Part model, mm, in its own coordinate system. A direction names the side the tool comes from. Give positions to 0.01 mm unless a question says otherwise; leave off trailing zeros. Loops run counter-clockwise (first coordinate to the right, second up) from the corner with the lowest first, then second, coordinate; pieces in that order, holes last. Notation, with made-up numbers: M 35,73 L 54,73 A24 ccw 54,84 Z; hole C 11,45.25 d4. An arc over 180 degrees is marked long. Answer in a Markdown table with one row per item.
Autodesk Inventor part; units mm, degrees
ref_plane "YZ Plane" through (0, 0, 0) normal (1, 0, 0) x (0, 1, 0)
ref_plane "XZ Plane" through (0, 0, 0) normal (0, 1, 0) x (-1, 0, 0)
ref_plane "XY Plane" through (0, 0, 0) normal (0, 0, 1) x (1, 0, 0)
sketch "Sketch1" plane through (0, 0, 0) normal (0, 0, 1) x (1, 0, 0)
  line L0 (0, 0) -> (-9.9, 0)
  line L1 (-9.9, 0) -> (-9.9, 10)
  line L2 (-9.9, 10) -> (0, 10)
  line L3 (0, 10) -> (0, 0)
  dimension "d0" = 9.9
  dimension "d1" = 10
extrude "Extrusion1" add sketch "Sketch1" along normal blind 9.9
sketch "Sketch2" plane through (0, 0, 0) normal (1, 0, 0) x (0, 0, -1)
  circle A0 centre (-5, 5) radius 2
  line L0 (0, 0) -> (-9.9, 0)
  line L1 (0, 0) -> (0, 10)
  point P0 (-4.95, 0)
  dimension "d4" = 4
  dimension "d5" = 5
  dimension "d6" = 5
extrude "Extrusion2" cut sketch "Sketch2" against normal blind 10
sketch "Sketch3" plane through (-9.9, 10, 0) normal (0, 1, 0) x (1, 0, 0)
  line L0 (0, 0) -> (0, -9.9)
  circle A0 centre (4.95, -4.95) radius 7.0004
  line L1 (9.9, 0) -> (0, 0)
  line L2 (-2.0504, -11.9504) -> (11.9504, -11.9504)
  line L3 (11.9504, -11.9504) -> (11.9504, 2.0504)
  line L4 (11.9504, 2.0504) -> (-2.0504, 2.0504)
  line L5 (-2.0504, 2.0504) -> (-2.0504, -11.9504)
  point P0 (-2.0504, -4.95)
  point P1 (4.95, 2.0504)
  point P2 (4.95, -11.9504)
  point P3 (11.9504, -4.95)
  dimension "d9" = 4.95
  dimension "d10" = 4.95
extrude "Extrusion3" add sketch "Sketch3" along normal blind 3
sketch "Sketch14" plane through (-9.9, 13, 0) normal (0, 1, 0) x (1, 0, 0)
  line L0 (-35.05, -80.9496) -> (44.95, -80.9496)
  line L1 (44.95, -80.9496) -> (44.95, 2.0504)
  line L2 (44.95, 2.0504) -> (-35.05, 2.0504)
  line L3 (-35.05, 2.0504) -> (-35.05, -80.9496)
  line L4 (11.9504, 2.0504) -> (-2.0504, 2.0504)
  line L5 (-35.05, 2.0504) -> (-38.05, 2.0504)
  line L6 (-38.05, 2.0504) -> (-38.05, -80.9496)
  line L7 (-38.05, -80.9496) -> (-35.05, -80.9496)
  line L8 (-35.05, -80.9496) -> (-35.05, 2.0504)
  line L9 (44.95, -80.9496) -> (47.95, -80.9496)
  line L10 (47.95, -80.9496) -> (47.95, 2.0504)
  line L11 (47.95, 2.0504) -> (44.95, 2.0504)
  line L12 (44.95, 2.0504) -> (44.95, -80.9496)
  point P0 (9.9, 0)
  point P1 (-35.05, -39.4496)
  point P2 (4.95, 2.0504)
  point P3 (4.95, 2.0504)
  point P4 (44.95, 2.0504)
  dimension "d60" = 40
  dimension "d61" = 40
  dimension "d62" = 0
  dimension "d63" = 83
  dimension "d64" = 3
  dimension "d65" = 3
  dimension "d68" = 83
extrude "Extrusion14" add sketch "Sketch14" along normal blind 3
sketch "Sketch15" plane through (-9.9, 16, 0) normal (0, 1, 0) x (1, 0, 0)
  line L0 (-2.0504, 2.0504) -> (-38.05, 2.0504)
  line L1 (-38.05, -80.9496) -> (47.95, -80.9496)
  line L2 (-38.05, 2.0504) -> (-35.05, 2.0504)
  line L3 (-35.05, 2.0504) -> (-35.05, -80.9496)
  line L4 (-35.05, -80.9496) -> (-38.05, -80.9496)
  line L5 (-38.05, -80.9496) -> (-38.05, 2.0504)
  line L6 (47.95, -80.9496) -> (47.95, 2.0504)
  line L7 (47.95, 2.0504) -> (44.95, 2.0504)
  line L8 (44.95, 2.0504) -> (44.95, -80.9496)
  line L9 (44.95, -80.9496) -> (47.95, -80.9496)
  line L10 (47.95, -80.9496) -> (47.95, 2.0504)
  line L11 (-38.05, 2.0504) -> (47.95, 2.0504)
  line L12 (47.95, 2.0504) -> (47.95, -0.9496)
  line L13 (47.95, -0.9496) -> (-38.05, -0.9496)
  line L14 (-38.05, -0.9496) -> (-38.05, 2.0504)
  point P0 (9.9, 0)
  point P1 (-35.05, -0.9496)
  point P2 (44.95, -0.9496)
  dimension "d69" = 3
  dimension "d70" = 3
  dimension "d71" = 3
extrude "Extrusion15" add sketch "Sketch15" along normal blind 14 contours L11 L8 L13 L3 L0 | L3 L13 L5 L0 | L7 L6 L13 L8 | L3 L1 L5 L13 | L13 L6 L1 L8
sketch "Sketch16" plane through (-9.9, 30, 0) normal (0, 1, 0) x (1, 0, 0)
  line L0 (47.95, 2.0504) -> (-38.05, 2.0504)
  line L1 (47.95, -80.9496) -> (47.95, 2.0504)
  line L2 (-38.05, 2.0504) -> (47.95, 2.0504)
  line L3 (47.95, 2.0504) -> (47.95, -80.9496)
  line L4 (47.95, -80.9496) -> (-38.05, -80.9496)
  line L5 (-38.05, -80.9496) -> (-38.05, 2.0504)
  point P0 (9.9, 0)
extrude "Extrusion16" add sketch "Sketch16" along normal blind 3
sketch "Sketch17" plane through (-9.9, 13, 0) normal (0, -1, 0) x (1, 0, 0)
  line L0 (39.95, 75.9496) -> (-30.05, 75.9496)
  line L1 (-30.05, 75.9496) -> (-30.05, 17.9496)
  line L2 (-30.05, 17.9496) -> (39.95, 17.9496)
  line L3 (39.95, 17.9496) -> (39.95, 75.9496)
  line L4 (47.95, -2.0504) -> (11.9504, -2.0504)
  line L5 (44.95, 80.9496) -> (44.95, 0.9496)
  line L6 (-38.05, 80.9496) -> (47.95, 80.9496)
  line L7 (-35.05, 0.9496) -> (-35.05, 80.9496)
  line L8 (36.95, 17.9496) -> (-30.05, 72.9496)
  line L9 (39.95, 20.9496) -> (-27.05, 75.9496)
  point P0 (9.9, 0)
  dimension "d76" = 20
  dimension "d77" = 5
  dimension "d78" = 5
  dimension "d79" = 5
  dimension "d88" = 3
  dimension "d89" = 3
  dimension "d90" = 3
extrude "Extrusion17" cut sketch "Sketch17" against normal blind 33 contours L3 L9 L0 | L8 L2 L1
sketch "Sketch18" plane through (38.05, 13, 80.9496) normal (1, 0, 0) x (0, 0, -1)
  line L0 (5, 12) -> (75, 12)
  line L1 (75, 12) -> (75, 8)
  line L2 (75, 8) -> (5, 8)
  line L3 (5, 8) -> (5, 12)
  line L4 (80, 17) -> (0, 17)
  line L5 (0, 3) -> (80, 3)
  line L6 (80, 3) -> (80, 17)
  line L7 (0, 0) -> (0, 20)
  point P0 (80.9496, -13)
  point P1 (80, 10)
  point P2 (75, 10)
  point P3 (0, 10)
  point P4 (5, 10)
  dimension "d82" = 5
  dimension "d83" = 5
  dimension "d84" = 5
  dimension "d85" = 5
extrude "Extrusion18" cut sketch "Sketch18" against normal blind 333 contours L0 L1 L2 L3
properties part number "shot_glass_tray"
(1) Drill centre lines: line 1 along Y through (x, z) = (-7, 5); line 2 along Y through (x, z) = (-0.5, 2); line 3 along Z through (x, y) = (-35.5, 14). Where is each one in solid material? Low to high.
Recorded:
| item | result |
|---|---|
| line 1 | y = 0 to 3, 7 to 16, 30 to 33 |
| line 2 | y = 0 to 16, 30 to 33 |
| line 3 | z = -2.05 to 17.95, 69.3 to 74.76, 75.95 to 80.95 |
(2) Saw through at D-D (y = 5). Write the cut outline in (x, z), plus the area to 3 significant figures.
Recorded:
| item | result |
|---|---|
| outline | M -9.9,0 L 0,0 L 0,3 L -9.9,3 Z; M -9.9,7 L 0,7 L 0,9.9 L -9.9,9.9 Z |
| area | 58.4 mm^2 |
(3) Pull direction Y, two halves, no side cores. Call faces 6 (the face through (4, 33, 39)), 7 (the face through (37, 21, 40)), 8 (the face through (35.05, 20, 40)), 9 (the face through (-3, 14, 75.95)): +Y half, -Y half, draft (parallel to the pull), parting line (faces both ways), or undercut.
Recorded:
| item | result |
|---|---|
| face 6 | +Y half |
| face 7 | undercut |
| face 8 | undercut |
| face 9 | draft |
(4) Saw through at B-B (z = 4.5). Write the cut outline in (x, y), plus the area to 3 significant figures.
Recorded:
| item | result |
|---|---|
| outline | M -47.95,13 L -11.95,13 L -11.95,10 L -9.9,10 L -9.9,6.94 L 0,6.94 L 0,10 L 2.05,10 L 2.05,13 L 38.05,13 L 38.05,33 L -47.95,33 Z; M -9.9,0 L 0,0 L 0,3.06 L -9.9,3.06 Z; hole M -44.95,16 L 35.05,16 L 35.05,30 L -44.95,30 Z |
| area | 703 mm^2 |
(5) Which spindle directions (+Z, -Z, +X, -X, +Y, -Y) get a long thin tool onto all of the face, cutting with end or side? Do faces 1 (the face through (-47.95, 20.6, 40)), 2 (the face through (37, 23, 75.95)), 3 (the face through (4, 30, 41)), 4 (the face through (2.05, 11, 5)), 5 (the face through (-2.981, 31.479, 48.065)). Say none if no direction does.
Recorded:
| item | result |
|---|---|
| face 1 | +Z, -Z, -X, +Y, -Y |
| face 2 | +X, -X |
| face 3 | +Z |
| face 4 | +Z, -Z, +X, -Y |
| face 5 | +Y, -Y |
(6) Pin check, flat tips, straight feed: pin 1 Ø12 at (x, z) = (28.5, 37.5) entering from -Y; pin 2 Ø0.9 at (y, z) = (11.5, 4.5) entering from -X; pin 3 Ø11 at (x, y) = (-6, 3) entering from -Z. Stop position of each tip, or through.
Recorded:
| item | result |
|---|---|
| pin 1 | stops at y = 13 |
| pin 2 | stops at x = -11.95 |
| pin 3 | stops at z = 0 |
(7) Saw through at A-A (y = 22). Write the cut outline in (x, z).
Recorded:
| item | result |
|---|---|
| outline | M -47.95,-2.05 L 38.05,-2.05 L 38.05,5.95 L 35.05,5.95 L 35.05,0.95 L -44.95,0.95 L -44.95,5.95 L -47.95,5.95 Z; M -47.95,75.95 L -44.95,75.95 L -44.95,80.95 L -47.95,80.95 Z; M 35.05,75.95 L 38.05,75.95 L 38.05,80.95 L 35.05,80.95 Z |
(8) Saw through at C-C (x = -30). Write the cut outline in (y, z), plus the area to 3 significant figures.
Recorded:
| item | result |
|---|---|
| outline | M 13,-2.05 L 33,-2.05 L 33,17.95 L 30,17.95 L 30,0.95 L 16,0.95 L 16,17.95 L 13,17.95 Z; M 13,64.78 L 16,64.78 L 16,70.24 L 13,70.24 Z; M 13,75.95 L 16,75.95 L 16,80.95 L 13,80.95 Z; M 30,64.78 L 33,64.78 L 33,70.24 L 30,70.24 Z; M 30,75.95 L 33,75.95 L 33,80.95 L 30,80.95 Z |
| area | 225 mm^2 |
